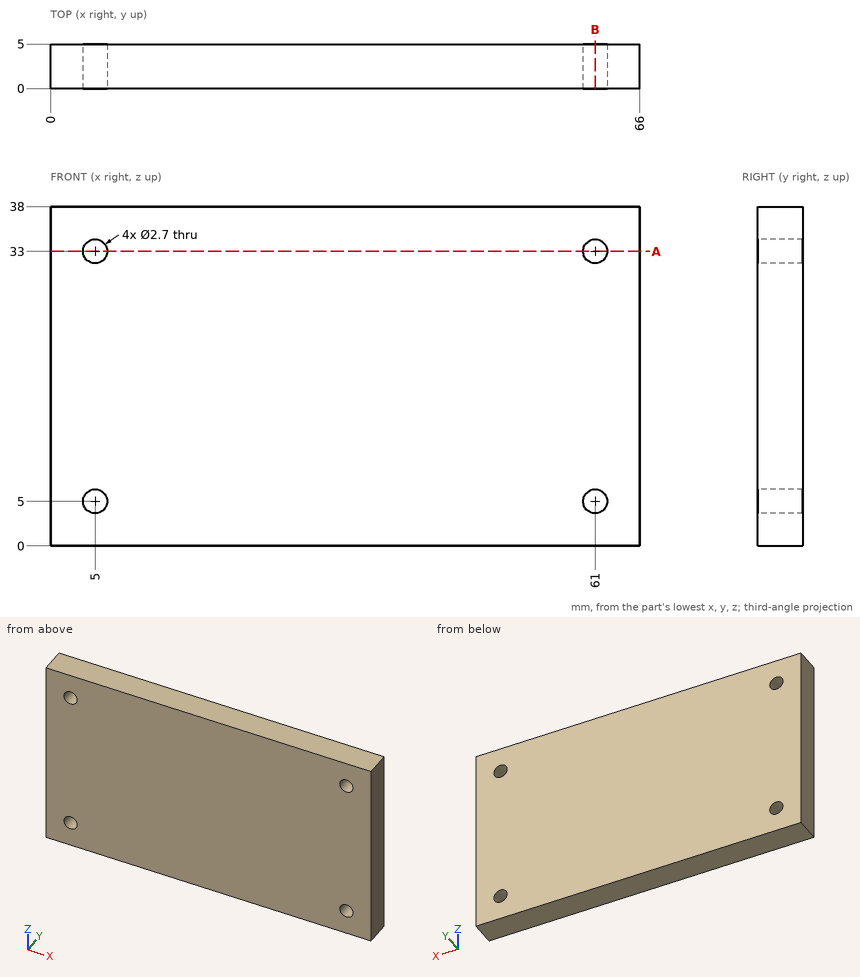
Job drawing, mm, ordinate dimensions from the low corner. One solid piece. Round coordinates to 2 decimals unless told otherwise and drop trailing zeros. Loops run counter-clockwise (first coordinate to the right, second up) from the corner with the lowest first, then second, coordinate; pieces in that order, holes last. Notation, with made-up numbers: (83.25, -20) -> (132.25, -20) arc R18 ccw to (132.25, -2) -> close; hole circle Ø2 at (-38, 89.25). An arc over 180 degrees is marked (long way). One line per item, written item: value. Start each with the question number.
Q1. Cut at B-B on x = 61. List the corners of the cut face in (y, z), plus the area to 3 significant figures.
Q2. Probe line 1 along Z through (x, y) = (5, 3.3); line 2 along X through (y, z) = (2.3, 32). List the from-to ranges inside material, lowest first.
Q3. Cut at A-A on z = 33. List the corners of the cut face in (x, y).
Q4. Drop flat-ended pins along their axis: pin 1 Ø1 at (x, y) = (58.5, 1.5) entering from -Z; pin 2 Ø1.6 at (x, z) = (61, 33) entering from +Y. Give the stop position or say it passes through.
Computed:
1. outline: (0, 0) -> (5, 0) -> (5, 3.65) -> (0, 3.65) -> close; (0, 6.35) -> (5, 6.35) -> (5, 31.65) -> (0, 31.65) -> close; (0, 34.35) -> (5, 34.35) -> (5, 38) -> (0, 38) -> close
1. area: 163 mm²
2. line 1: 0 to 3.65, 6.35 to 31.65, 34.35 to 38
2. line 2: 0 to 4.09, 5.91 to 60.09, 61.91 to 66
3. outline: (0, 0) -> (3.65, 0) -> (3.65, 5) -> (0, 5) -> close; (6.35, 0) -> (59.65, 0) -> (59.65, 5) -> (6.35, 5) -> close; (62.35, 0) -> (66, 0) -> (66, 5) -> (62.35, 5) -> close
4. pin 1: z = 0
4. pin 2: through
